Geometry check sheet. Reference: the model listing, model coordinates, mm. Face numbers are marked on the shaded views. A direction names the side the tool comes from. Round coordinates to 2 decimals unless told otherwise and drop trailing zeros. Order: outer loops, then holes, each group sorted by start corner. A loop starts at its lowest first (then second) coordinate and runs counter-clockwise, first axis right, second up.
(1) Sectioned sample at A-A (z = 31). Record the boundary of the cut face in (x, y).
(2) Set-up check for the marked faces 1 and 2: record each of +Z, -Z, +X, -X, +Y, -Y from which the full face is reachable in a straight line by a thin tool's end or side.
(3) Release check for a two-part mould opening along X. For the marked faces 3 and 4 record: +X half, -X half, draft (parallel to the pull), parting line (faces both ways), or undercut.
(4) Go/stop test with flat-tipped pins: pin 1 (2 mm diameter, centred on x = -12, y = -12, fed in from +Z); pin 2 (3 mm diameter, centred on x = -12.5, z = 27.5, fed in from -Y); pin 3 (8 mm diameter, centred on y = -1, z = 13, fed in from +X). Record where each tip stops, or that it passes through.
(5) Material ranges on line 1 along Y through (x, z) = (0, 16.5); line 2 along X through (y, z) = (-13.5, 28); line 3 along Y through (x, z) = (17, 43), recorded low to high.
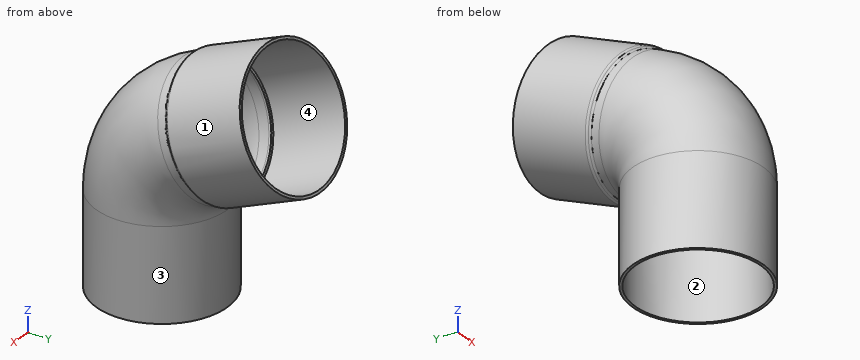
from build123d import *

# Parameters (mm, degrees)
ESQUISSE6_R        = 25
ESQUISSE6_R_2      = 24
ESQUISSE8_R        = 26
ESQUISSE8_R_2      = 24
EXTRU_MINCE1_DEPTH = 1
EXTRU_MINCE2_START = 30
ESQUISSE9_R        = 26
ESQUISSE9_R_2      = 25
EXTRU_MINCE2_DEPTH = 30
CONG_1_R           = 1
CONG_2_R           = 1


with BuildPart() as part:
    # Balayage-Mince2: sweep along a path in Esquisse7
    with BuildLine(Plane(origin=(0, 0, 0), x_dir=(0, 0, -1), z_dir=(1, 0, 0))) as balayage_mince2_path:
        Line((0, 0), (-35.14343316412919, -3.47e-15))
        ThreePointArc((-35.14343316412919, -3.47e-15), (-51.70154272349097, 4.983425337984965), (-62.75857876770245, 18.27806614532184))
        Line((-62.75857876770245, 18.27806614532184), (-64.37754708374251, 22.092116482858586))
    # Esquisse6 → Balayage-Mince2 (sweep)
    with BuildSketch(Plane.XY):
        Circle(ESQUISSE6_R)
        Circle(ESQUISSE6_R_2, mode=Mode.SUBTRACT)
    sweep(path=balayage_mince2_path.line)



with BuildPart() as body_2:
    # Esquisse8 → Extru.-Mince1 (new body)
    with BuildSketch(Plane(origin=(0, 41.87396099217143, 17.77444189612002), x_dir=(1, 0, 0), z_dir=(0, 0.9205048534524412, 0.39073112848927183))):
        with Locations((0, -50.62776693988426)):
            Circle(ESQUISSE8_R)
        with Locations((0, -50.62776693988426)):
            Circle(ESQUISSE8_R_2, mode=Mode.SUBTRACT)
    extrude(amount=EXTRU_MINCE1_DEPTH)


with BuildPart() as part_1:
    add(part.part)

    add(body_2.part)  # Extru.-Mince2 merges body 2
    # Esquisse9 → Extru.-Mince2 (add)
    with BuildSketch(Plane(origin=(0, 42.794465845623876, 18.16517302460929), x_dir=(1, 0, 0), z_dir=(0, 0.9205048534524412, 0.39073112848927183)).offset(EXTRU_MINCE2_START)):
        with Locations((0, -50.627766939884246)):
            Circle(ESQUISSE9_R)
        with Locations((0, -50.627766939884246)):
            Circle(ESQUISSE9_R_2, mode=Mode.SUBTRACT)
    extrude(amount=-EXTRU_MINCE2_DEPTH)

    # Congé1
    cong_1_edges = [part_1.edges().sort_by_distance(p)[0] for p in [
        (-25, 22.09211648285859, 64.3775470837425),
    ]]
    fillet(cong_1_edges, radius=CONG_1_R - 0.0001)  # a hair under: the kernel refuses the full size

    # Congé2
    cong_2_edges = [part_1.edges().sort_by_distance(p)[0] for p in [
        (-26, 22.092116482858604, 64.37754708374253),
    ]]
    fillet(cong_2_edges, radius=CONG_2_R)


solid = part_1.part
Answer below:
1. outline: circle Ø50 at (0, 0); hole circle Ø48 at (0, 0)
2. face 1: none
2. face 2: -Z
3. face 3: parting line
3. face 4: undercut
4. pin 1: stops at z = 67.28
4. pin 2: stops at y = -22.45
4. pin 3: stops at x = 25
5. line 1: y = -25 to -24, 24 to 25
5. line 2: x = -21.04 to -19.84, 19.84 to 21.04
5. line 3: y = -17.69 to -16.28, 19.57 to 21.37
